Build history of the part. All positions in model axes, mm. Face numbers are marked on the shaded views. A direction names the side the tool comes from. Give positions to 0.01 mm unless a question says otherwise; leave off trailing zeros. Write each loop counter-clockwise with the first axis right and the second up, starting at its lowest first coordinate (ties: lowest second). Pieces come first, ordered by that corner, then holes.
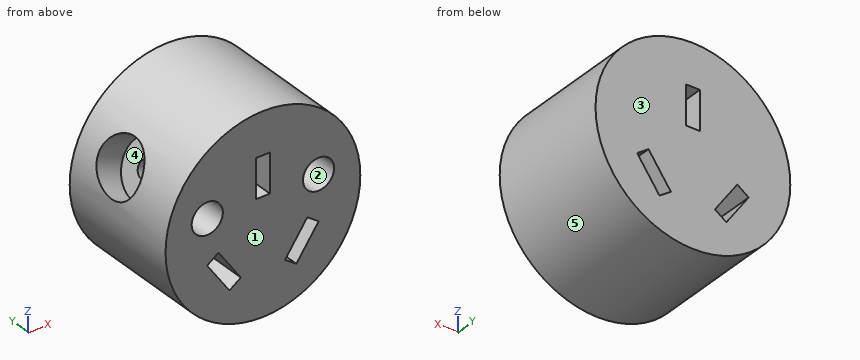
from build123d import *

# Parameters (mm, degrees)
SALIENTE_EXTRUIR1_DEPTH      = 11.5
SALIENTE_EXTRUIR1_DEPTH_BACK = 11.5
CROQUIS1_R                   = 17.5
CROQUIS2_W                   = 2.5
CROQUIS2_H                   = 7
CORTAR_EXTRUIR_L_MINA1_DEPTH = 34.786091813
TALADRO2_D                   = 5.6
TALADRO2_DEPTH               = 7
TALADRO3_D                   = 3
TALADRO3_DEPTH               = 15
TALADRO3_CBORE_D             = 10
TALADRO3_CBORE_DEPTH         = 5


with BuildPart() as part:
    # Croquis1 → Saliente-Extruir1 (new, two sides: drawn at the far end of the back side and taken through both)
    with BuildSketch(Plane(origin=(0, 0, 0), x_dir=(1, 0, 0), z_dir=(0, 1, 0)).offset(-SALIENTE_EXTRUIR1_DEPTH_BACK)):
        with Locations(Location((0, 0, 0), (0, 0, 270))):
            Circle(CROQUIS1_R)
    extrude(amount=SALIENTE_EXTRUIR1_DEPTH + SALIENTE_EXTRUIR1_DEPTH_BACK)

    # Croquis2 → Cortar-Extruir-L_mina1 (cut, through all)
    with BuildSketch(Plane(origin=(0, 11.5, 0), x_dir=(1, 0, 0), z_dir=(0, 1, 0))):
        with Locations((0, -6.5)):
            Rectangle(CROQUIS2_W, CROQUIS2_H)
        Polygon((-7.976059945, 3.548965145), (-3.96102489, 9.283029455), (-6.008905001, 10.716970545), (-10.023940055, 4.982906235), align=None)
        Polygon((3.96102489, 9.283029455), (7.976059945, 3.548965145), (10.023940055, 4.982906235), (6.008905001, 10.716970545), align=None)
    extrude(amount=-CORTAR_EXTRUIR_L_MINA1_DEPTH, mode=Mode.SUBTRACT)

    # Taladro2
    with Locations(Plane(origin=(0, -11.5, 0), x_dir=(-1, 0, 0), z_dir=(0, -1, 0))):
        with Locations((-10, -3), (10, -3)):
            Hole(TALADRO2_D / 2, depth=TALADRO2_DEPTH)

    # Taladro3
    with Locations(Plane(origin=(-15.907017578, 1.665123618, 7.294984015), x_dir=(-0.416856229443, 0, -0.908972433011), z_dir=(-0.908972433011, 0, 0.416856229443))):
        with Locations((0, 0)):
            CounterBoreHole(TALADRO3_D / 2, TALADRO3_CBORE_D / 2, TALADRO3_CBORE_DEPTH, depth=TALADRO3_DEPTH)


solid = part.part
1. Drill centre lines: line 1 along Z through (x, y) = (-9, -7.5); line 2 along X through (y, z) = (-6.25, 0.5); line 3 along X through (y, z) = (1.75, -6). Where is each one in solid material? Low to high.
2. Mould opens along X. For the marked faces 3, 4 and 5 say: pulls with the +X half, pulls with the -X half, needs draft (parallel to the pull), parting line crosses it, or undercut.
3. Saw through at C-C on y = -1.25. Give the cut face in (x, z).
4. Saw through at B-B on x = 0. Give the cut face in (y, z), plus the area to 3 significant figures.
5. Drop flat-ended pins along their axis: pin 1 (8 mm diameter, centred on y = 3, z = -8.5, fed in from +X); pin 2 (4 mm diameter, centred on x = -10, y = -1, fed in from -Z); pin 3 (3 mm diameter, centred on y = 5.5, z = 4, fed in from -X). Give the stop position or say it passes through.
6. 3-axis set-ups, long thin cutter, end or side, ignore diameter. For the marked faces 1 and 2: which of +Z, -Z, +X, -X, +Y, -Y reach the whole face in a straight line?
7. Saw through at A-A on y = -7.75. Give the cut face in (x, z).
8. Saw through at D-D on z = -4.5. Give the cut face in (x, y), plus the area to 3 significant figures.
Outcome:
1. line 1: z = -15.01 to -6.45, -4.27 to 0.38, 5.62 to 15.01
1. line 2: x = -17.49 to -11.26, -8.74 to 8.74, 11.26 to 17.49
1. line 3: x = -16.44 to -9.31, -6.26 to 6.26, 9.31 to 16.44
2. face 3: needs draft
2. face 4: undercut
2. face 5: parting line crosses it
3. outline: (-17.17, 3.4) arc R17.5 ccw (long way) to (-13.78, 10.79) - (-9.67, 8.9) - (-13.06, 1.52) - close; hole (-10.02, -4.98) - (-6.01, -10.72) - (-3.96, -9.28) - (-7.98, -3.55) - close; hole (-1.25, 3) - (1.25, 3) - (1.25, 10) - (-1.25, 10) - close; hole (3.96, -9.28) - (6.01, -10.72) - (10.02, -4.98) - (7.98, -3.55) - close
4. outline: (-11.5, -17.5) - (11.5, -17.5) - (11.5, 3) - (-11.5, 3) - close; (-11.5, 10) - (11.5, 10) - (11.5, 17.5) - (-11.5, 17.5) - close
4. area: 644 mm2
5. pin 1: stops at x = 16.91
5. pin 2: stops at z = -15.56
5. pin 3: stops at x = -17.32
6. face 1: +Z, -Z, +X, -X, -Y
6. face 2: -Y
7. outline: circle Ø35 at (0, 0); hole circle Ø5.6 at (-10, 3); hole (-10.02, -4.98) - (-6.01, -10.72) - (-3.96, -9.28) - (-7.98, -3.55) - close; hole (-1.25, 3) - (1.25, 3) - (1.25, 10) - (-1.25, 10) - close; hole (3.96, -9.28) - (6.01, -10.72) - (10.02, -4.98) - (7.98, -3.55) - close; hole circle Ø5.6 at (10, 3)
8. outline: (-16.91, -11.5) - (-9.33, -11.5) - (-9.33, 11.5) - (-16.91, 11.5) - close; (-7.31, -11.5) - (7.31, -11.5) - (7.31, 11.5) - (-7.31, 11.5) - close; (9.33, -11.5) - (16.91, -11.5) - (16.91, 11.5) - (9.33, 11.5) - close
8. area: 685 mm2
